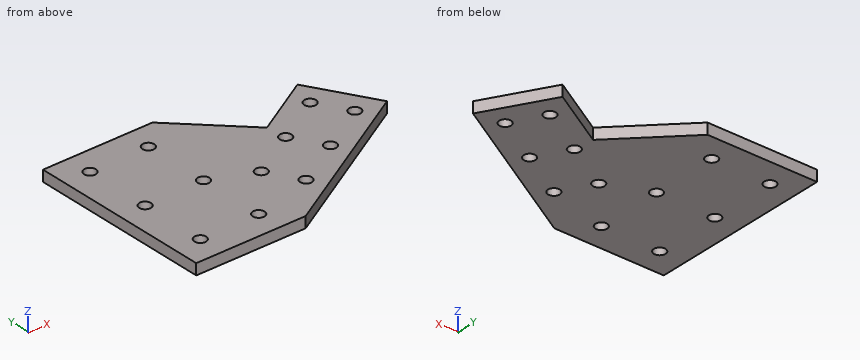
from build123d import *

# Parameters (mm, degrees)
EXTRUDE_1_DEPTH     = 3
SKETCH_2_R          = 1.6
CUT_EXTRUDE_1_DEPTH = 67.211781429


with BuildPart() as part:
    # 草图1 → 凸台-拉伸1 (new body)
    with BuildSketch(Plane.XY):
        Polygon((0, 0), (-30, 0), (-30, 50), (0, 50), (17.057713659, 32.942286341), (33.301270189, 42.320508076), (43.301270189, 25), align=None)
    extrude(amount=EXTRUDE_1_DEPTH)

    # 草图2 → 切除-拉伸1 (cut, through all)
    with BuildSketch(Plane.XY.offset(3)):
        with Locations((-23, 43)):
            Circle(SKETCH_2_R)
        with Locations((-7, 43)):
            Circle(SKETCH_2_R)
        with Locations((-23, 7)):
            Circle(SKETCH_2_R)
        with Locations((-7, 7)):
            Circle(SKETCH_2_R)
        with Locations((-23, 25)):
            Circle(SKETCH_2_R)
        with Locations((-7, 25)):
            Circle(SKETCH_2_R)
        with Locations((30.605117767, 34.990381057)):
            Circle(SKETCH_2_R)
        with Locations((35.605117767, 26.330127019)):
            Circle(SKETCH_2_R)
        with Locations((22.61473671, 18.830127019)):
            Circle(SKETCH_2_R)
        with Locations((17.61473671, 27.490381057)):
            Circle(SKETCH_2_R)
        with Locations((4.624355653, 19.990381057)):
            Circle(SKETCH_2_R)
        with Locations((9.624355653, 11.330127019)):
            Circle(SKETCH_2_R)
    extrude(amount=-CUT_EXTRUDE_1_DEPTH, mode=Mode.SUBTRACT)


solid = part.part
Here's how the part is built. I have some questions about the finished solid (model axes, mm). Round coordinates to 2 decimals unless told otherwise and drop trailing zeros. Order: outer loops, then holes, each group sorted by start corner. A loop starts at its lowest first (then second) coordinate and runs counter-clockwise, first axis right, second up. Notation, with made-up numbers: (-24, 75) -> (9, 75) arc R7 ccw to (9, 79) -> close; hole circle Ø8 at (57.25, -1.75). An arc over 180 degrees is marked (long way). Use CSV: the item, a comma, the result in double quotes.
1. I need wall thicknesses on line 1 along Y through (x, z) = (-23, 0.9); line 2 along X through (y, z) = (34, 0.75); line 3 along X through (y, z) = (27, 2.8). Which ranges of each line are inside material? Lowest first, please.
Recorded:
line 1,"y = 0 to 5.4, 8.6 to 23.4, 26.6 to 41.4, 44.6 to 50"
line 2,"x = -30 to 16, 18.89 to 29.35, 31.86 to 38.11"
line 3,"x = -30 to 16.09, 19.14 to 34.15, 37.06 to 42.15"
2. I want a section at B-B on y = 7. List the corners of the cut face in (x, z) for me, and give its area (3 significant figures).
Recorded:
outline,"(-30, 0) -> (-24.6, 0) -> (-24.6, 3) -> (-30, 3) -> close; (-21.4, 0) -> (-8.6, 0) -> (-8.6, 3) -> (-21.4, 3) -> close; (-5.4, 0) -> (12.12, 0) -> (12.12, 3) -> (-5.4, 3) -> close"
area,"107 mm2"
3. I want a section at D-D on x = 23. List the corners of the cut face in (y, z) for me.
Recorded:
outline,"(13.28, 0) -> (17.28, 0) -> (17.28, 3) -> (13.28, 3) -> close; (20.38, 0) -> (36.37, 0) -> (36.37, 3) -> (20.38, 3) -> close"
4. I'm going to push flat-ended pins straight in: P1, Ø1.9, axis at x = 4.62, y = 19.99, coming from the +Z side; P2, Ø1.5, axis at y = 21.5, z = 2.5, coming from the +X side. Where does each tip first touch, or does it pass through?
Recorded:
P1,"passes through"
P2,"stops at x = 38.54"
5. I want a section at A-A on x = -7. List the corners of the cut face in (y, z) for me, and give its area (3 significant figures).
Recorded:
outline,"(0, 0) -> (5.4, 0) -> (5.4, 3) -> (0, 3) -> close; (8.6, 0) -> (23.4, 0) -> (23.4, 3) -> (8.6, 3) -> close; (26.6, 0) -> (41.4, 0) -> (41.4, 3) -> (26.6, 3) -> close; (44.6, 0) -> (50, 0) -> (50, 3) -> (44.6, 3) -> close"
area,"121 mm2"
6. I want a section at C-C on z = 0.9. Give the number of separate pieces and of enclosed holes in the cut face, and give its area (3 significant figures).
Recorded:
separate pieces,"1"
enclosed holes,"12"
area,"2,520 mm2"
